Answer from the drawing. Dimensions are ordinates in mm from the lowest x, y and z of the part. Give positions to 0.01 mm unless a question says otherwise; leave off trailing zeros. Order: outer loops, then holes, each group sorted by start corner. A loop starts at its lowest first (then second) coordinate and runs counter-clockwise, first axis right, second up. Notation, with made-up numbers: (3, 80) - (31, 80) arc R23 ccw to (31, 99) - close; hole circle Ø9 at (41, 65.5). An arc over 180 degrees is marked (long way). One line per item, written item: value. Start each with the question number.
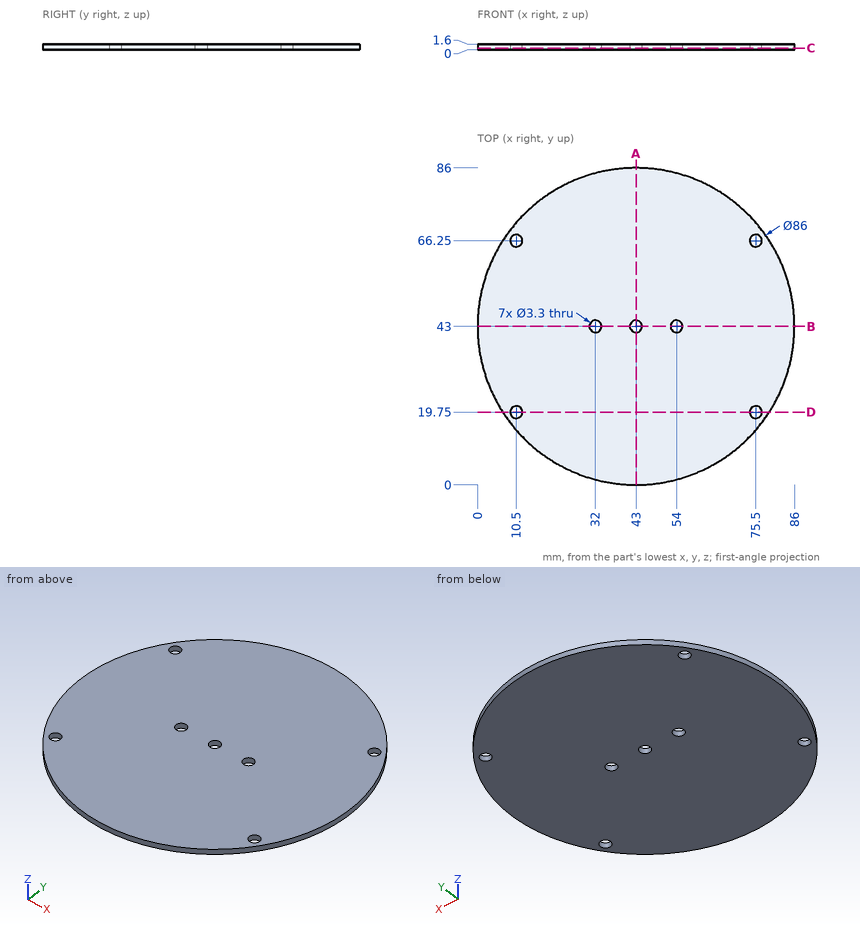
1) Find the intervals of material crossed by probe 1 along Y at (x, z) = (75.5, 1); probe 2 along X at (y, z) = (66.25, 0.8); probe 3 along X at (y, z) = (67, 1.5), in increasing order. Write a range as from..to.
2) Section A-A on x = 43 is taken. Write down the section's boundary in (y, z).
3) This flat-tipped pin is pushed along its axis until it touches: pin 1 (2 mm diameter, centred on x = 75.5, y = 19.75, fed in from -Z). Where does it stop, or does it pass through?
4) Section D-D on y = 19.75 is taken. Write down the section's boundary in (x, z), plus the area to 3 significant figures.
5) Section B-B on y = 43 is taken. Write down the section's boundary in (x, z).
6) Section C-C on z = 0.5 is taken. Write down the section's boundary in (x, y), plus the area to 3 significant figures.
Solved:
1. probe 1: y = 14.84..18.1, 21.4..64.6, 67.9..71.16
1. probe 2: x = 6.83..8.85, 12.15..73.85, 77.15..79.17
1. probe 3: x = 7.32..9.03, 11.97..74.03, 76.97..78.68
2. outline: (0, 0) - (41.35, 0) - (41.35, 1.6) - (0, 1.6) - close; (44.65, 0) - (86, 0) - (86, 1.6) - (44.65, 1.6) - close
3. pin 1: passes through
4. outline: (6.83, 0) - (8.85, 0) - (8.85, 1.6) - (6.83, 1.6) - close; (12.15, 0) - (73.85, 0) - (73.85, 1.6) - (12.15, 1.6) - close; (77.15, 0) - (79.17, 0) - (79.17, 1.6) - (77.15, 1.6) - close
4. area: 105 mm2
5. outline: (0, 0) - (30.35, 0) - (30.35, 1.6) - (0, 1.6) - close; (33.65, 0) - (41.35, 0) - (41.35, 1.6) - (33.65, 1.6) - close; (44.65, 0) - (52.35, 0) - (52.35, 1.6) - (44.65, 1.6) - close; (55.65, 0) - (86, 0) - (86, 1.6) - (55.65, 1.6) - close
6. outline: circle Ø86 at (43, 43); hole circle Ø3.3 at (10.5, 19.75); hole circle Ø3.3 at (10.5, 66.25); hole circle Ø3.3 at (32, 43); hole circle Ø3.3 at (43, 43); hole circle Ø3.3 at (54, 43); hole circle Ø3.3 at (75.5, 19.75); hole circle Ø3.3 at (75.5, 66.25)
6. area: 5,750 mm2
